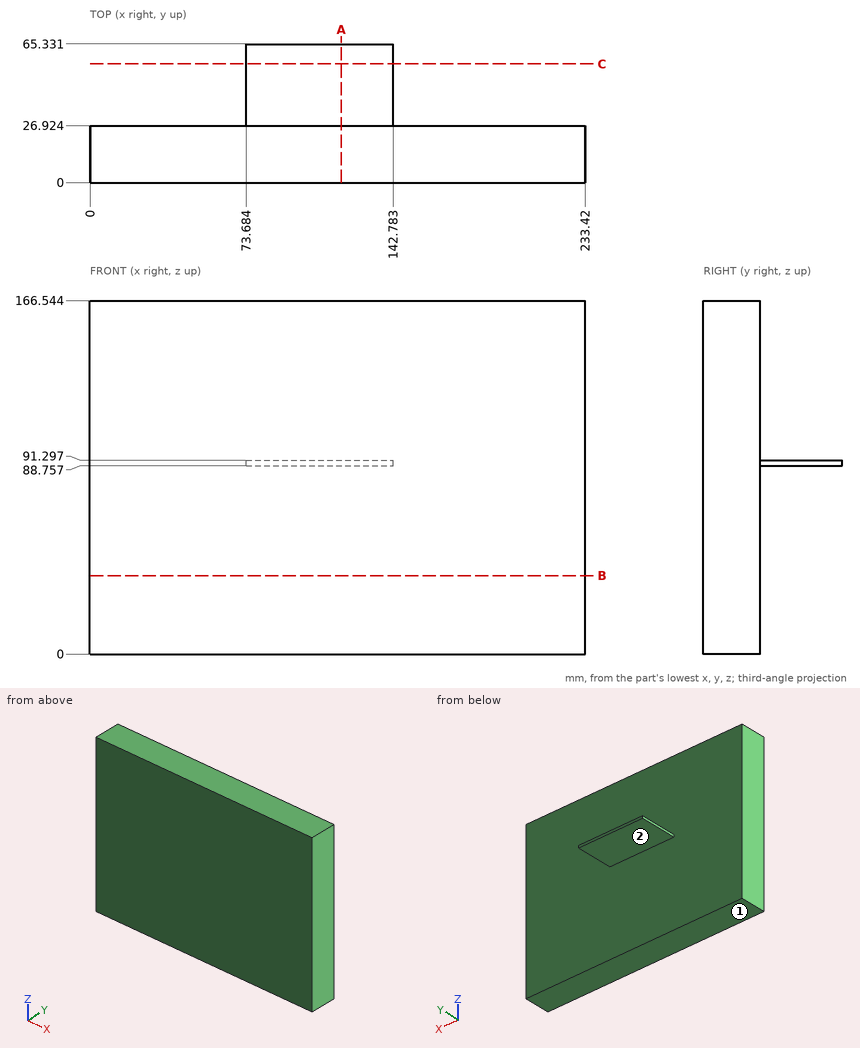
Geometry: see drawing. Coordinates: mm, zero at the bounding-box minimum. A direction names the side the tool comes from. Coordinates: 2 decimals unless noted, no trailing zeros. Loops run counter-clockwise (first coordinate to the right, second up) from the corner with the lowest first, then second, coordinate; pieces in that order, holes last. Notation, with made-up numbers: (19, -23) - (68, -23) arc R21 ccw to (68, 8) - close; hole circle Ø3 at (54, -5). An arc over 180 degrees is marked (long way). Return JSON: item names as keys, results as strings.
Q1. Contact query for flat-ended pins moving along their axis: P1, Ø12, axis at x = 145.5, z = 45.5, coming from the +Y side; P2, Ø0.8, axis at y = 46.5, z = 89.5, coming from the +X side; P3, Ø2, axis at x = 126.5, y = 37.5, coming from the -Z side. Output: stop coordinate, or through.
Results:
{"P1": "y = 26.92", "P2": "x = 142.78", "P3": "z = 88.76"}
Q2. Material intervals for line 1 along Y through (x, z) = (151.5, 25); line 2 along Z through (x, y) = (139, 50), sorted ascending.
Results:
{"line 1": "0 to 26.92", "line 2": "88.76 to 91.3"}
Q3. Section B-B, the plane z = 37. Return loops of the section in (x, y).
Results:
{"outline": "(0, 0) - (233.42, 0) - (233.42, 26.92) - (0, 26.92) - close"}
Q4. Section C-C, the plane y = 56. Return loops of the section in (x, z).
Results:
{"outline": "(73.68, 88.76) - (142.78, 88.76) - (142.78, 91.3) - (73.68, 91.3) - close"}
Q5. Access query for the marked faces 1 and 2. Directions: +Z, -Z, +X, -X, +Y, -Y. A direction counts if a zero-diameter tool reaches every point of the face in a straight line with its end or side. Return the directions, or none.
Results:
{"face 1": "-Z, +X, -X, +Y, -Y", "face 2": "-Z, +X, -X, +Y"}
Q6. Section A-A, the plane x = 118.5. Return loops of the section in (y, z), plus the area to 3 significant figures.
Results:
{"outline": "(0, 0) - (26.92, 0) - (26.92, 88.76) - (65.33, 88.76) - (65.33, 91.3) - (26.92, 91.3) - (26.92, 166.54) - (0, 166.54) - close", "area": "4,580 mm2"}
